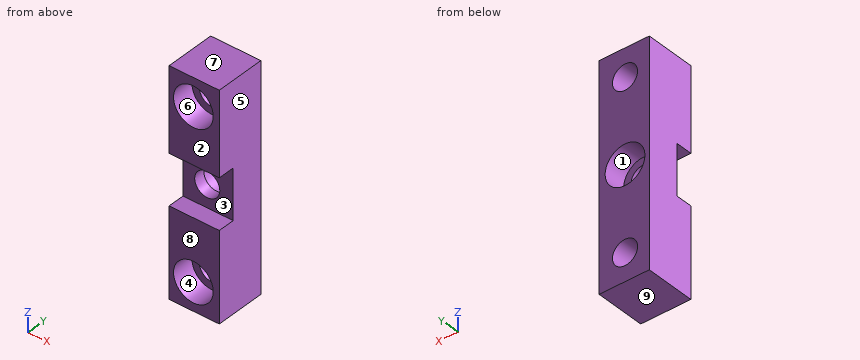
from build123d import *

# Parameters (mm, degrees)
F0_W           = 18
F0_H           = 80
F1_DEPTH       = 18
F3_D           = 9
F3_DEPTH       = 18.75
F3_CBORE_D     = 14.25
F3_CBORE_DEPTH = 8
F3_TIP         = 2.7038727856
F4_W           = 18
F4_H           = 18
F5_DEPTH       = 6
F7_D           = 9
F7_DEPTH       = 18.75
F7_CBORE_D     = 14.25
F7_CBORE_DEPTH = 8
F7_TIP         = 2.7038727856


with BuildPart() as f1:
    # F0 (on Front) → F1 (new body)
    with BuildSketch(Plane.XZ):
        with Locations((0.2960520796, 4.8042173386)):
            Rectangle(F0_W, F0_H)
    extrude(amount=F1_DEPTH)

    # F3
    with Locations(Plane.XZ.offset(18)):
        with Locations((0, 34.8042173386), (0, -25.1957826614)):
            CounterBoreHole(F3_D / 2, F3_CBORE_D / 2, F3_CBORE_DEPTH, depth=F3_DEPTH)
            with Locations((0, 0, -(F3_DEPTH + F3_TIP / 2))):  # 118° drill point
                Cone(0, F3_D / 2, F3_TIP, mode=Mode.SUBTRACT)

    # F4 (on face) → F5 (cut)
    with BuildSketch(Plane.XZ.offset(18)):
        with Locations((0.2960520796, 5.8042173386)):
            Rectangle(F4_W, F4_H)
    extrude(amount=-F5_DEPTH, mode=Mode.SUBTRACT)

    # F7
    with Locations(Plane(origin=(0, 0, 0), x_dir=(-1, 0, 0), z_dir=(0, 1, 0))):
        with Locations((0, 4.8042173386)):
            CounterBoreHole(F7_D / 2, F7_CBORE_D / 2, F7_CBORE_DEPTH, depth=F7_DEPTH)
            with Locations((0, 0, -(F7_DEPTH + F7_TIP / 2))):  # 118° drill point
                Cone(0, F7_D / 2, F7_TIP, mode=Mode.SUBTRACT)


solid = f1.part
Input: part model. Units: mm. Frame: model coordinates. Face numbers are marked on the shaded views. A direction names the side the tool comes from. Coordinates: 2 decimals unless noted, no trailing zeros. Loops run counter-clockwise (first coordinate to the right, second up) from the corner with the lowest first, then second, coordinate; pieces in that order, holes last. Notation, with made-up numbers: (-1, -26) -> (49, -26) arc R16 cw to (49, 0) -> close; hole circle Ø8 at (-28.5, 2). An arc over 180 degrees is marked (long way). One line per item, written item: value.
(1) Draft query along Z for the marked faces 6, 7, 8 and 9. Return one class per face: pulls with the +Z half, pulls with the -Z half, needs draft (parallel to the pull), parting line crosses it, or undercut.
Answer below:
face 6: undercut
face 7: pulls with the +Z half
face 8: needs draft
face 9: pulls with the -Z half
(2) Pin query (flat end, axial travel): pin 1 Ø8.5 at (x, z) = (0, 4.8) entering from +Y. Return the tip coordinate at first contact, or that it passes through.
Answer below:
pin 1: passes through
(3) Ray query, line 1 along Z through (x, y) = (0, -2); line 2 along Z through (x, y) = (0, -9.75); line 3 along Y through (x, z) = (3.75, -21.5). Return the intervals inside material, ascending.
Answer below:
line 1: z = -35.2 to -29.7, -20.7 to -2.32, 11.93 to 30.3, 39.3 to 44.8
line 2: z = -35.2 to -29.7, -20.7 to 0.3, 9.3 to 30.3, 39.3 to 44.8
line 3: y = -10 to 0
(4) Set-up query: the marked faces 1, 2, 3, 4 and 5. Return all of +Z, -Z, +X, -X, +Y, -Y with unobstructed straight access to the full face (end or side cutting, diameter ignored); none if empty.
Answer below:
face 1: +Y
face 2: +Z, -Z, +X, -X, -Y
face 3: +X, -X, -Y
face 4: -Y
face 5: +Z, -Z, +X, +Y, -Y
(5) Cut plane B-B (z = 38). Output: boundary loops of the cut face in (x, y).
Answer below:
outline: (-8.7, -18) -> (-6.37, -18) -> (-6.37, -10) -> (-3.17, -10) -> (-3.17, 0) -> (-8.7, 0) -> close; (3.17, -10) -> (6.37, -10) -> (6.37, -18) -> (9.3, -18) -> (9.3, 0) -> (3.17, 0) -> close
(6) Cut plane D-D (z = 11). Output: boundary loops of the cut face in (x, y).
Answer below:
outline: (-8.7, -12) -> (9.3, -12) -> (9.3, 0) -> (3.52, 0) -> (3.52, -8) -> (-3.52, -8) -> (-3.52, 0) -> (-8.7, 0) -> close
(7) Cut plane A-A (x = 0). Give the number of separate pieces and of enclosed holes in the cut face, then the cut area to 3 significant figures.
Answer below:
separate pieces: 4
enclosed holes: 0
area: 774 mm2
(8) Cut plane C-C (z = -19.5). Output: boundary loops of the cut face in (x, y).
Answer below:
outline: (-8.7, -18) -> (-4.28, -18) -> (-4.28, -10) -> (4.28, -10) -> (4.28, -18) -> (9.3, -18) -> (9.3, 0) -> (-8.7, 0) -> close
